from build123d import *

# Parameters (mm, degrees)
SKETCH1_R           = 5
BOSS_EXTRUDE1_DEPTH = 50
CHAMFER1_SIZE       = 1
CUT_EXTRUDE1_START  = -2.5
SKETCH2_R           = 6
SKETCH2_R_2         = 4
CUT_EXTRUDE1_DEPTH  = 1
CUT_EXTRUDE2_START  = -3.5
SKETCH3_R           = 5
SKETCH3_R_2         = 4
CUT_EXTRUDE2_DEPTH  = 1


with BuildPart() as part:
    # Sketch1 → Boss-Extrude1 (new body)
    with BuildSketch(Plane(origin=(0, 0, 0), x_dir=(1, 0, 0), z_dir=(0, 1, 0))):
        with Locations(Location((0, 0, 0), (0, 0, 270))):
            Circle(SKETCH1_R)
    extrude(amount=BOSS_EXTRUDE1_DEPTH)

    # Chamfer1
    chamfer1_edges = [part.edges().sort_by_distance(p)[0] for p in [
        (0, 0, -5),
        (0, 50, -5),
    ]]
    chamfer(chamfer1_edges, length=CHAMFER1_SIZE)

    # Sketch2 → Cut-Extrude1 (cut)
    with BuildSketch(Plane.XZ.offset(CUT_EXTRUDE1_START)):
        Circle(SKETCH2_R)
        with Locations(Location((0, 0, 0), (0, 0, 270))):
            Circle(SKETCH2_R_2, mode=Mode.SUBTRACT)
    extrude(amount=-CUT_EXTRUDE1_DEPTH, mode=Mode.SUBTRACT)

    # Sketch3 → Cut-Extrude2 (cut)
    with BuildSketch(Plane(origin=(0, 50, 0), x_dir=(1, 0, 0), z_dir=(0, 1, 0)).offset(CUT_EXTRUDE2_START)):
        with Locations(Location((0, 0, 0), (0, 0, 90))):
            Circle(SKETCH3_R)
        with Locations(Location((0, 0, 0), (0, 0, 90))):
            Circle(SKETCH3_R_2, mode=Mode.SUBTRACT)
    extrude(amount=CUT_EXTRUDE2_DEPTH, mode=Mode.SUBTRACT)


solid = part.part
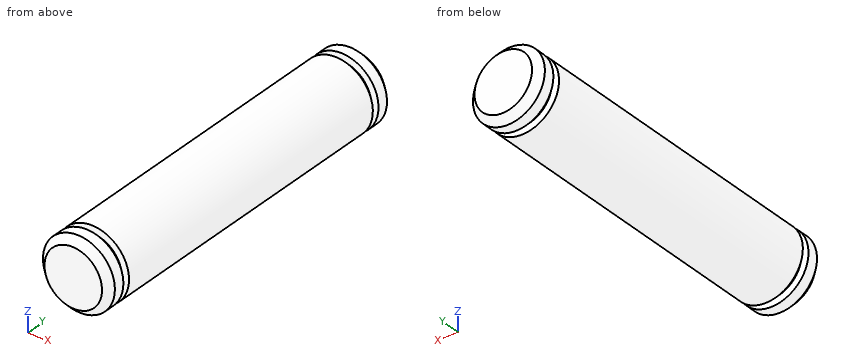
CAD build for the part. Positions are in the model's coordinates, mm. Coordinates: 2 decimals unless noted, no trailing zeros. Write each loop counter-clockwise with the first axis right and the second up, starting at its lowest first coordinate (ties: lowest second). Pieces come first, ordered by that corner, then holes. Notation, with made-up numbers: M 23,20 L 58,20 A26 ccw 58,52 Z; hole C 64,65 d8. An arc over 180 degrees is marked long. Answer as a JSON object with one key per item and string values. Group by question number.
1) Pin check, flat tips, straight feed: pin 1 Ø4 at (x, y) = (-0.5, 9.5) entering from -Z; pin 2 Ø3 at (x, y) = (3.5, 13.5) entering from +Z; pin 3 Ø2 at (y, z) = (31.5, 2) entering from +X; pin 4 Ø3 at (y, z) = (28.5, -2.5) entering from -X. Stop position of each tip, or through.
2) Wall check: line 1 (Y direction, x = -2.25, z = 4); line 2 (Y direction, x = -3.25, z = 3); line 3 (X direction, y = 21, z = -0.25). Give the ranges that are in metal, low to high. Write a range as from..to.
3) Saw through at A-A (y = 10.5). Write the cut outline in (x, z), plus the area to 3 significant figures.
Values follow:
{
 "1": {"pin 1": "stops at z = -5", "pin 2": "stops at z = 4.58", "pin 3": "stops at x = 4.9", "pin 4": "stops at x = -4.9"},
 "2": {"line 1": "y = 0.59..2.5, 3.5..46.5, 47.5..49.41", "line 2": "y = 0.42..2.5, 3.5..46.5, 47.5..49.58", "line 3": "x = -4.99..4.99"},
 "3": {"outline": "C 0,0 d10", "area": "78.5 mm2"}
}
